Verification items for the finished model (mm, model axes). A direction names the side the tool comes from. Coordinates: 2 decimals unless noted, no trailing zeros. Write each loop counter-clockwise with the first axis right and the second up, starting at its lowest first coordinate (ties: lowest second). Pieces come first, ordered by that corner, then holes. Notation, with made-up numbers: (42.5, 89) -> (58.5, 89) arc R24 cw to (58.5, 116) -> close; hole circle Ø3 at (56.5, -29.75). An arc over 180 degrees is marked (long way). Answer in a Markdown table with one row per item.
Autodesk Inventor part; units mm, degrees
ref_plane "YZ Plane" through (0, 0, 0) normal (1, 0, 0) x (0, 1, 0)
ref_plane "XZ Plane" through (0, 0, 0) normal (0, 1, 0) x (-1, 0, 0)
ref_plane "XY Plane" through (0, 0, 0) normal (0, 0, 1) x (1, 0, 0)
sketch "Sketch1" plane through (0, 0, 0) normal (1, 0, 0) x (0, 1, 0)
  line L0 (0, 0) -> (50.8, 0)
  line L1 (50.8, 0) -> (50.8, -25.4)
  line L2 (50.8, -25.4) -> (0, -25.4)
  line L3 (0, -25.4) -> (0, 0)
  line L4 (47.625, -3.175) -> (3.175, -3.175)
  line L5 (3.175, -3.175) -> (3.175, -22.225)
  line L6 (3.175, -22.225) -> (47.625, -22.225)
  line L7 (47.625, -22.225) -> (47.625, -3.175)
  dimension "d0" = 50.8
  dimension "d1" = 25.4
  dimension "d2" = 3.175
extrude "Extrusion1" add sketch "Sketch1" along normal blind 98.425
sketch "Sketch2" plane through (0, 0, -25.4) normal (0, 0, -1) x (-1, 0, 0)
  line L0 (0, 50.8) -> (-98.425, 50.8)
  line L1 (0, 50.8) -> (0, 0)
  line L2 (0, 0) -> (-98.425, 0)
  point P0 (-22.225, 25.4)
  dimension "d5" = 25.4
  dimension "d6" = 22.225
hole "Hole2" at (22.225, 25.4, -25.4) direction (0, 0, 1) diameter 15.875 end through all
sketch "Sketch3" plane through (0, 0, -25.4) normal (0, 0, -1) x (-1, 0, 0)
  circle A0 centre (-85.725, 12.7) radius 3.175
  circle A1 centre (-60.325, 41.275) radius 3.175
  line L0 (0, 0) -> (-98.425, 0)
  line L1 (-98.425, 0) -> (-98.425, 50.8)
  dimension "d23" = 6.35
  dimension "d24" = 6.35
  dimension "d25" = 12.7
  dimension "d26" = 38.1
  dimension "d27" = 41.275
  dimension "d28" = 12.7
extrude "Extrusion2" cut sketch "Sketch3" against normal blind 25.4
properties part number "15102898-16-P-0304" material "Aluminum 6061"
1. Section check D-D, the plane x = 75.5. Record the boundary of the cut face in (y, z) (3 decimals).
Geometry says:
| item | result |
|---|---|
| outline | (0, -25.4) -> (50.8, -25.4) -> (50.8, 0) -> (0, 0) -> close; hole (3.175, -22.225) -> (47.625, -22.225) -> (47.625, -3.175) -> (3.175, -3.175) -> close |
2. Section check B-B, the plane z = -9.25. Record the boundary of the cut face in (x, y) (3 decimals), plus the area to 3 significant figures.
Geometry says:
| item | result |
|---|---|
| outline | (0, 0) -> (98.425, 0) -> (98.425, 3.175) -> (0, 3.175) -> close; (0, 47.625) -> (98.425, 47.625) -> (98.425, 50.8) -> (0, 50.8) -> close |
| area | 625 mm^2 |
3. Tool access check on faces 1 (the flat face through (49, 3.175, -13)), 2 (the cylindrical face through (88.245, 10.768, -23.835)). Record the directions out of +Z, -Z, +X, -X, +Y, -Y that give a thin tool (end or side, any length) a straight path to the whole face; none if there is none.
Geometry says:
| item | result |
|---|---|
| face 1 | +X, -X |
| face 2 | +Z, -Z |
4. Section check A-A, the plane y = 25.4. Record the boundary of the cut face in (x, z) (1 decimal), plus the area to 3 significant figures.
Geometry says:
| item | result |
|---|---|
| outline | (0, -25.4) -> (14.3, -25.4) -> (14.3, -22.2) -> (0, -22.2) -> close; (0, -3.2) -> (14.3, -3.2) -> (14.3, 0) -> (0, 0) -> close; (30.2, -25.4) -> (98.4, -25.4) -> (98.4, -22.2) -> (30.2, -22.2) -> close; (30.2, -3.2) -> (98.4, -3.2) -> (98.4, 0) -> (30.2, 0) -> close |
| area | 524 mm^2 |
5. Depth check by flat-ended pin: P1, Ø6, axis at y = 32, z = -5.5, coming from the +X side (3 decimals); P2, Ø5, axis at x = 60.325, y = 41.275, coming from the -Z side. Enter the tip coordinate at first touch or a pass-through.
Geometry says:
| item | result |
|---|---|
| P1 | x = 98.425 |
| P2 | through |
6. Thickness scan on line 1 (Y direction, x = 7.5, z = -3.5) (3 decimals); line 2 (Z direction, x = 74, y = 29.5) (3 decimals); line 3 (X direction, y = 25.4, z = -22.95) (1 decimal). Record the ranges inside material, lowest first. Write a range as from..to.
Geometry says:
| item | result |
|---|---|
| line 1 | 0..3.175, 47.625..50.8 |
| line 2 | -25.4..-22.225, -3.175..0 |
| line 3 | 0..14.3, 30.2..98.4 |
7. Section check C-C, the plane y = 34.5. Record the boundary of the cut face in (x, z) (3 decimals).
Geometry says:
| item | result |
|---|---|
| outline | (0, -25.4) -> (98.425, -25.4) -> (98.425, -22.225) -> (0, -22.225) -> close; (0, -3.175) -> (98.425, -3.175) -> (98.425, 0) -> (0, 0) -> close |
8. Mould release check, pull along Z, two halves, no side actions. Record for faces 3 (the flat face through (49, 26, -3.175)), 4 (the flat face through (49, 25, 0)), 5 (the cylindrical face through (88.245, 10.768, -1.61)): released by +Z, released by -Z, zero draft, split by the parting line, or undercut.
Geometry says:
| item | result |
|---|---|
| face 3 | undercut |
| face 4 | released by +Z |
| face 5 | zero draft |
